Part model, mm, in its own coordinate system. A direction names the side the tool comes from. Round coordinates to 2 decimals unless told otherwise and drop trailing zeros. Loops run counter-clockwise (first coordinate to the right, second up) from the corner with the lowest first, then second, coordinate; pieces in that order, holes last. Notation, with made-up numbers: (7, 18) -> (26, 18) arc R25 cw to (26, 43) -> close; hole circle Ø1 at (-9, 55.25). An arc over 180 degrees is marked (long way). Use a Markdown table: item, result. Add a question column.
Item 1: Cut at C-C, the plane z = 6.75. State how many separate pieces and enclosed holes the cut face has, plus the area to 3 significant figures.
Item 2: Cut at A-A, the plane y = 17. List the corners of the cut face in (x, z).
Item 3: Probe line 1 (X direction, y = 19, z = 2.25); line 2 (X direction, y = 17.25, z = 14); line 3 (Y direction, x = -31.75, z = 19). List the from-to ranges inside material, lowest first. Write a range as [from, to].
Item 4: Flat gauge pins, fed straight in: pin 1 (0.5 mm diameter, centred on x = -24, y = 18, fed in from -Z); pin 2 (1.1 mm diameter, centred on x = -32.5, y = 16, fed in from +Z). Where does each tip first touch, or does it go through?
Item 5: Cut at D-D, the plane y = 16. List the corners of the cut face in (x, z), plus the area to 3 significant figures.
Item 6: Cut at B-B, the plane x = -31.5. List the corners of the cut face in (y, z).
Item 7: Two-plate mould, pull along Y, no slides. Class faces 4 (the face through (-37.635, 14.752, 10.799)), 5 (the face through (-35.369, 20.366, 16.37)), 6 (the face through (-30, 18, 21.3)): pulls with the +Y half, pulls with the -Y half, needs draft (parallel to the pull), parting line crosses it, or undercut.
Item 8: Which spindle directions (+Z, -Z, +X, -X, +Y, -Y) get a long thin tool onto all of the face, cutting with end or side? Do faces 1 (the face through (-24, 18, 3.5)), 2 (the face through (-31.77, 20, 8)), 3 (the face through (-30.571, 20.366, 16.37)). Say none if no direction does.
```python
from build123d import *

# Parameters (mm, degrees)
F0_W     = 8
F0_H     = 7
F1_DEPTH = 3.5
F2_W     = 8
F2_H     = 7
F2_W_2   = 4.4
F2_H_2   = 3.4
F3_DEPTH = 3
F4_W     = 8
F4_H     = 7
F5_DEPTH = 3.5
F6_W     = 16
F6_H     = 7
F6_W_2   = 4.4
F6_H_2   = 3.4
F7_DEPTH = 1.3
F8_W     = 16
F8_H     = 7
F9_DEPTH = 10
F10_R    = 1
F11_R    = 1


with BuildPart() as f1:
    # F0 (on Top) → F1 (new body)
    with BuildSketch(Plane.XY):
        with Locations((-33.920105, 17.951032)):
            Rectangle(F0_W, F0_H)
        Polygon((-34.470105, 19.451032), (-30.470105, 19.451032), (-30.470105, 16.451032), (-34.470105, 16.451032), (-34.470105, 17.451032), (-36.470105, 17.451032), (-36.470105, 18.451032), (-34.470105, 18.451032), align=None, mode=Mode.SUBTRACT)
        Polygon((-29.370105, 21.451032), (-29.920105, 21.451032), (-29.920105, 14.451032), (-21.920105, 14.451032), (-21.920105, 21.451032), (-23.370105, 21.451032), (-25.370105, 21.451032), align=None)
        Polygon((-29.370105, 16.451032), (-29.370105, 19.451032), (-25.370105, 19.451032), (-25.370105, 18.451032), (-23.370105, 18.451032), (-23.370105, 17.451032), (-25.370105, 17.451032), (-25.370105, 16.451032), align=None, mode=Mode.SUBTRACT)
    extrude(amount=F1_DEPTH)

    # F2 (on face) → F3 (join)
    with BuildSketch(Plane.XY.offset(3.5)):
        with Locations((-33.920105, 17.951032)):
            Rectangle(F2_W, F2_H)
        with Locations((-32.470105, 17.951032)):
            Rectangle(F2_W_2, F2_H_2, mode=Mode.SUBTRACT)
        with Locations((-25.920105, 17.951032)):
            Rectangle(F2_W, F2_H)
        with Locations((-27.370105, 17.951032)):
            Rectangle(F2_W_2, F2_H_2, mode=Mode.SUBTRACT)
    extrude(amount=F3_DEPTH)

    # F4 (on face) → F5 (join)
    with BuildSketch(Plane.XY.offset(6.5)):
        with Locations((-25.920105, 17.951032)):
            Rectangle(F4_W, F4_H)
        Polygon((-28.070105, 19.651032), (-28.070105, 20.651032), (-27.370105, 20.651032), (-26.670105, 20.651032), (-26.670105, 19.651032), (-25.170105, 19.651032), (-25.170105, 16.251032), (-26.670105, 16.251032), (-26.670105, 15.251032), (-27.370105, 15.251032), (-28.070105, 15.251032), (-28.070105, 16.251032), (-29.570105, 16.251032), (-29.570105, 19.651032), align=None, mode=Mode.SUBTRACT)
        with Locations((-33.920105, 17.951032)):
            Rectangle(F4_W, F4_H)
        Polygon((-34.670105, 17.951032), (-34.670105, 19.651032), (-33.170105, 19.651032), (-33.170105, 20.651032), (-32.470105, 20.651032), (-31.770105, 20.651032), (-31.770105, 19.651032), (-30.270105, 19.651032), (-30.270105, 17.951032), (-30.270105, 16.251032), (-31.770105, 16.251032), (-31.770105, 15.251032), (-32.470105, 15.251032), (-33.170105, 15.251032), (-33.170105, 16.251032), (-34.670105, 16.251032), align=None, mode=Mode.SUBTRACT)
    extrude(amount=F5_DEPTH)

    # F6 (on face) → F7 (join)
    with BuildSketch(Plane.XY.offset(10)):
        with Locations((-29.920105, 17.951032)):
            Rectangle(F6_W, F6_H)
        with Locations((-32.470105, 17.951032)):
            Rectangle(F6_W_2, F6_H_2, mode=Mode.SUBTRACT)
        with Locations((-27.370105, 17.951032)):
            Rectangle(F6_W_2, F6_H_2, mode=Mode.SUBTRACT)
    extrude(amount=F7_DEPTH)

    # F8 (on face) → F9 (join)
    with BuildSketch(Plane.XY.offset(11.3)):
        with Locations((-29.920105, 17.951032)):
            Rectangle(F8_W, F8_H)
        Polygon((-30.270105, 20.651032), (-30.270105, 19.651032), (-30.270105, 16.251032), (-30.270105, 15.251032), (-35.670105, 15.251032), (-35.670105, 20.651032), align=None, mode=Mode.SUBTRACT)
        Polygon((-29.570105, 15.251032), (-29.570105, 16.251032), (-29.570105, 19.651032), (-29.570105, 20.651032), (-24.170105, 20.651032), (-24.170105, 15.251032), align=None, mode=Mode.SUBTRACT)
    extrude(amount=F9_DEPTH)

    # F10
    f10_edges = [f1.edges().sort_by_distance(p)[0] for p in [
        (-37.920105, 14.451032, 10.65),
        (-21.920105, 14.451032, 10.65),
        (-37.920105, 21.451032, 10.65),
        (-21.920105, 21.451032, 10.65),
    ]]
    fillet(f10_edges, radius=F10_R)

    # F11
    f11_edges = [f1.edges().sort_by_distance(p)[0] for p in [
        (-24.170105, 15.251032, 16.3),
        (-30.270105, 15.251032, 16.3),
        (-35.670105, 15.251032, 16.3),
        (-29.570105, 15.251032, 16.3),
        (-24.170105, 20.651032, 16.3),
        (-30.270105, 20.651032, 16.3),
        (-29.570105, 20.651032, 16.3),
        (-35.670105, 20.651032, 16.3),
    ]]
    fillet(f11_edges, radius=F11_R)


solid = f1.part
```
A:
| question | item | result |
|---|---|---|
| 1 | separate pieces | 1 |
| 1 | enclosed holes | 2 |
| 1 | area | 75.6 mm^2 |
| 2 | outline | (-37.92, 0) -> (-34.47, 0) -> (-34.47, 3.5) -> (-34.67, 3.5) -> (-34.67, 11.3) -> (-35.67, 11.3) -> (-35.67, 21.3) -> (-37.92, 21.3) -> close; (-30.47, 0) -> (-29.37, 0) -> (-29.37, 3.5) -> (-29.57, 3.5) -> (-29.57, 21.3) -> (-30.27, 21.3) -> (-30.27, 3.5) -> (-30.47, 3.5) -> close; (-25.37, 0) -> (-21.92, 0) -> (-21.92, 21.3) -> (-24.17, 21.3) -> (-24.17, 11.3) -> (-25.17, 11.3) -> (-25.17, 3.5) -> (-25.37, 3.5) -> close |
| 3 | line 1 | x = [-37.92, -34.47], [-30.47, -29.37], [-25.37, -21.92] |
| 3 | line 2 | x = [-37.92, -35.67], [-30.27, -29.57], [-24.17, -21.92] |
| 3 | line 3 | y = [14.45, 15.25], [20.65, 21.45] |
| 4 | pin 1 | stops at z = 3.5 |
| 4 | pin 2 | stops at z = 11.3 |
| 5 | outline | (-37.92, 0) -> (-21.92, 0) -> (-21.92, 21.3) -> (-24.2, 21.3) -> (-24.2, 11.3) -> (-29.54, 11.3) -> (-29.54, 21.3) -> (-30.3, 21.3) -> (-30.3, 11.3) -> (-35.64, 11.3) -> (-35.64, 21.3) -> (-37.92, 21.3) -> close; hole (-33.17, 6.5) -> (-31.77, 6.5) -> (-31.77, 10) -> (-33.17, 10) -> close; hole (-28.07, 6.5) -> (-26.67, 6.5) -> (-26.67, 10) -> (-28.07, 10) -> close |
| 5 | area | 224 mm^2 |
| 6 | outline | (14.45, 0) -> (16.45, 0) -> (16.45, 3.5) -> (16.25, 3.5) -> (16.25, 11.3) -> (15.25, 11.3) -> (15.25, 21.3) -> (14.45, 21.3) -> close; (19.45, 0) -> (21.45, 0) -> (21.45, 21.3) -> (20.65, 21.3) -> (20.65, 11.3) -> (19.65, 11.3) -> (19.65, 3.5) -> (19.45, 3.5) -> close |
| 7 | face 4 | pulls with the -Y half |
| 7 | face 5 | undercut |
| 7 | face 6 | needs draft |
| 8 | face 1 | -Z |
| 8 | face 2 | none |
| 8 | face 3 | +Z |
